Part print with two shaded views. Sizes in mm from the minimum x, y, z corner. A direction names the side the tool comes from. Coordinates: 2 decimals unless noted, no trailing zeros. Order: outer loops, then holes, each group sorted by start corner. A loop starts at its lowest first (then second) coordinate and runs counter-clockwise, first axis right, second up. Notation, with made-up numbers: (71.25, -7.5) - (124.25, -7.5) arc R7 ccw to (124.25, 3.5) - close; hole circle Ø3 at (55, -17.75). An arc over 180 degrees is marked (long way). One line per item, written item: value.
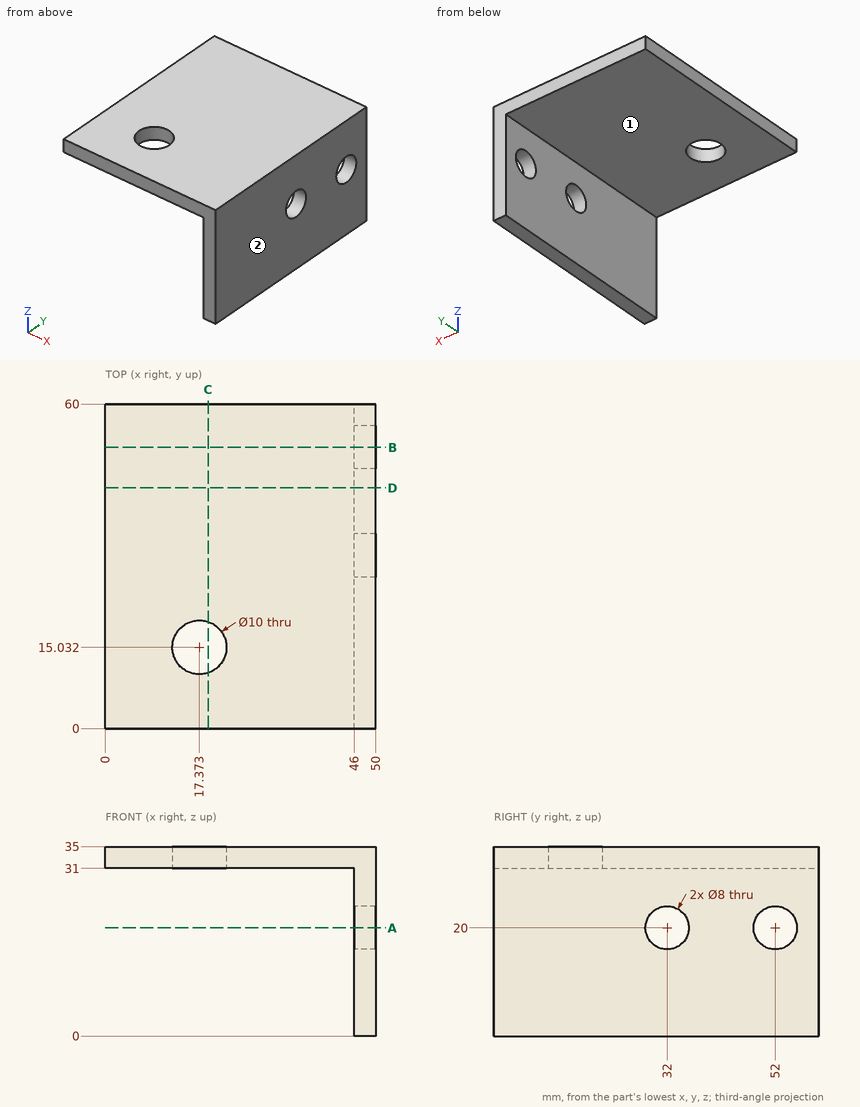
1. Flat gauge pin, fed straight in: P1, Ø5, axis at y = 32, z = 20, coming from the +X side. Where does the tip first touch, or does it go through?
Values found:
P1: passes through
2. Band-saw the part on D-D, the plane y = 44.5. Give the cut face in (x, z).
Values found:
outline: (0, 31) - (46, 31) - (46, 0) - (50, 0) - (50, 35) - (0, 35) - close
3. Band-saw the part on B-B, the plane y = 52. Give the cut face in (x, z), and give its area (3 significant figures).
Values found:
outline: (0, 31) - (46, 31) - (46, 24) - (50, 24) - (50, 35) - (0, 35) - close; (46, 0) - (50, 0) - (50, 16) - (46, 16) - close
area: 292 mm2
4. Band-saw the part on C-C, the plane x = 19. Give the cut face in (y, z), and give its area (3 significant figures).
Values found:
outline: (0, 31) - (10.3, 31) - (10.3, 35) - (0, 35) - close; (19.76, 31) - (60, 31) - (60, 35) - (19.76, 35) - close
area: 202 mm2
5. Probe line 1 along Y through (x, z) = (47.45, 20); line 2 along Z through (x, y) = (7, 33); line 3 along X through (y, z) = (42.5, 30). List the from-to ranges inside material, lowest first.
Values found:
line 1: y = 0 to 28, 36 to 48, 56 to 60
line 2: z = 31 to 35
line 3: x = 46 to 50
6. Band-saw the part on A-A, the plane z = 20. Give the cut face in (x, y).
Values found:
outline: (46, 0) - (50, 0) - (50, 28) - (46, 28) - close; (46, 36) - (50, 36) - (50, 48) - (46, 48) - close; (46, 56) - (50, 56) - (50, 60) - (46, 60) - close
7. 3-axis set-ups, long thin cutter, end or side, ignore diameter. For the marked faces 1 and 2: which of +Z, -Z, +X, -X, +Y, -Y reach the whole face in a straight line?
Values found:
face 1: -Z, -X, +Y, -Y
face 2: +Z, -Z, +X, +Y, -Y
